Autodesk Inventor part; units mm, degrees
ref_plane "YZ Plane" through (0, 0, 0) normal (1, 0, 0) x (0, 1, 0)
ref_plane "XZ Plane" through (0, 0, 0) normal (0, 1, 0) x (-1, 0, 0)
ref_plane "XY Plane" through (0, 0, 0) normal (0, 0, 1) x (1, 0, 0)
sketch "Sketch1" plane through (0, 0, 0) normal (0, 0, 1) x (1, 0, 0)
  line L0 (0, 0) -> (19.05, 0)
  line L1 (19.05, 0) -> (19.05, 19.05)
  line L2 (69.85, 19.05) -> (69.85, 0)
  line L3 (69.85, 0) -> (88.9, 0)
  line L4 (88.9, 0) -> (88.9, 38.1)
  line L5 (88.9, 38.1) -> (66.675, 57.15)
  line L6 (66.675, 57.15) -> (22.225, 57.15)
  line L7 (22.225, 57.15) -> (0, 38.1)
  line L8 (0, 38.1) -> (0, 0)
  arc A0 (69.85, 19.05) -> (19.05, 19.05) centre (44.45, 19.05) ccw
  dimension "d0" = 38.1
  dimension "d1" = 44.45
  dimension "d2" = 88.9
  dimension "d3" = 19.05
  dimension "d5" = 19.05
  dimension "d6" = 19.05
extrude "Extrusion1" add sketch "Sketch1" against normal blind 127
sketch "Sketch2" plane through (22.225, 57.15, 0) normal (0, 1, 0) x (1, 0, 0)
  line L0 (-22.225, 19.05) -> (68.7148, 19.05)
  line L1 (-22.225, 0) -> (-22.225, 127)
  line L2 (-22.225, 107.95) -> (68.7148, 107.95)
  line L3 (68.7148, 107.95) -> (68.7148, 19.05)
  line L4 (-22.225, 19.05) -> (-22.225, 107.95)
  line L5 (44.45, 0) -> (0, 0)
  line L6 (0, 127) -> (44.45, 127)
  dimension "d9" = 19.05
  dimension "d10" = 19.05
extrude "Extrusion2" cut sketch "Sketch2" against normal through all
sketch "Sketch3" plane through (88.9, 0, 0) normal (1, 0, 0) x (0, 0, -1)
  point P0 (0, 0)
sketch "Sketch4" plane through (88.9, 0, 0) normal (1, 0, 0) x (0, 0, -1)
  line L0 (0, 57.15) -> (0, 88.9)
  line L1 (25.4, 88.9) -> (25.4, 76.2)
  line L2 (25.4, 76.2) -> (101.6, 76.2)
  line L3 (101.6, 76.2) -> (101.6, 88.9)
  line L4 (101.6, 88.9) -> (127, 88.9)
  line L5 (127, 88.9) -> (127, 57.15)
  line L6 (127, 57.15) -> (0, 57.15)
  arc A0 (25.4, 88.9) -> (0, 88.9) centre (12.7, 88.9) ccw
  circle A1 centre (12.7, 88.9) radius 6.35
  point P0 (0, 0)
  dimension "d13" = 31.75
  dimension "d14" = 25.4
  dimension "d15" = 12.7
  dimension "d17" = 12.7
extrude "Extrusion3" add sketch "Sketch4" against normal blind 88.9
sketch "Sketch5" plane through (0, 0, 0) normal (0, 0, 1) x (1, 0, 0)
  line L0 (22.225, 104.8309) -> (22.225, 46.8186)
  line L1 (66.675, 46.8186) -> (66.6601, 105.2632)
  line L2 (0, 57.15) -> (0, 88.9)
  line L3 (22.225, 104.8309) -> (0, 104.8309)
  line L4 (0, 104.8309) -> (0, 57.15)
  line L5 (22.225, 57.15) -> (22.225, 104.8309)
  line L6 (66.6601, 105.2632) -> (88.8851, 105.2632)
  line L7 (88.8851, 105.2632) -> (88.8851, 57.15)
  line L8 (88.8851, 57.15) -> (66.675, 57.15)
  line L9 (0, 57.15) -> (22.225, 57.15)
  line L10 (22.225, 57.15) -> (0, 57.15)
  line L11 (88.9, 57.15) -> (66.675, 57.15)
  line L12 (66.6601, 105.2632) -> (88.9, 105.2632)
  line L13 (88.9, 105.2632) -> (88.9, 57.15)
  line L14 (88.9, 57.15) -> (66.6601, 57.15)
  line L15 (66.6601, 57.15) -> (66.6601, 105.2632)
  point P0 (0, 0)
  dimension "d20" = 22.225
  dimension "d21" = 44.45
extrude "Extrusion4" cut sketch "Sketch5" against normal through all
sketch "Sketch6" plane through (0, 0, 0) normal (0, 0, 1) x (1, 0, 0)
  line L0 (66.6601, 57.15) -> (22.225, 57.15)
  line L1 (34.925, 57.15) -> (34.925, 106.1689)
  line L2 (34.925, 106.1689) -> (53.975, 106.1689)
  line L3 (53.975, 106.1689) -> (53.975, 57.15)
  line L4 (22.225, 88.9) -> (22.225, 57.15)
  point P0 (0, 0)
  dimension "d24" = 19.05
  dimension "d25" = 12.7
extrude "Extrusion5" cut sketch "Sketch6" against normal through all
properties part number "HW 4 Part 4" material "Iron, Cast"
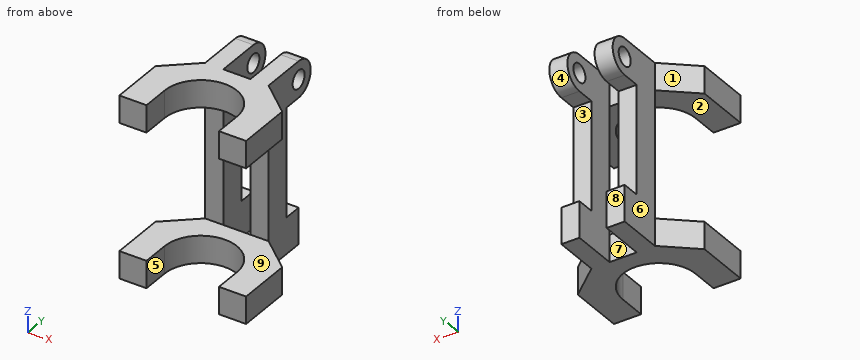
Work out the finished part from the listing and answer in its coordinate system (mm). Face numbers are marked on the shaded views. A direction names the side the tool comes from. Give positions to 0.01 mm unless a question says otherwise; leave off trailing zeros. Loops run counter-clockwise (first coordinate to the right, second up) from the corner with the lowest first, then second, coordinate; pieces in that order, holes last. Notation, with made-up numbers: (39.5, -28.5) -> (66.5, -28.5) arc R13 cw to (66.5, -9.5) -> close; hole circle Ø6 at (45, -33.75). An arc over 180 degrees is marked (long way). Put each result on its own line as item: value. Start each with the question number.
Item 1: The part is cut by section A-A (x = 44.45). Give the vertices of the cut face in (y, z), then the cut area to 3 significant figures.
Item 2: The part is cut by section D-D (y = 40). Give the vertices of the cut face in (x, z).
Item 3: The part is cut by section C-C (y = 74). Give the vertices of the cut face in (x, z) (3 decimals).
Item 4: Each of these flat-tipped pins is pushed along its axis until it touches: P1, Ø3, axis at x = 36, y = 40.5, coming from the +Z side; P2, Ø5, axis at y = 58, z = -108.5, coming from the -X side; P3, Ø1, axis at x = 63, z = -89.5, coming from the +Y side; P4, Ø3, axis at y = 70, z = -70, coming from the +X side. Where does it stop, or does it pass through?
Item 5: The mould has two halves that part along Z. Classify the marked faces 1, 2, 3 and 4: released by +Z, released by -Z, zero draft, split by the parting line, or undercut.
Item 6: The part is cut by section B-B (z = -12.7). Give the vertices of the cut face in (x, y) (3 decimals).
Item 7: Find the intervals of material crossed by L1, parallel to X at y = 92, z = -6.5 (3 decimals); L2, parallel to Z at x = 85, y = 16.5; L3, parallel to Z at x = 57, y = 88, in increasing order. Write a range as [from, to].
Item 8: Which of the six approach directions +Z, -Z, +X, -X, +Y, -Y give full straight-line access (tool end or side, diameter ignored) to the marked faces 5, 6, 7, 8 and 9?
Answers below:
1. outline: (44.45, -127) -> (57.15, -127) -> (57.15, -107.95) -> (44.45, -107.95) -> close; (44.45, -19.05) -> (57.15, -19.05) -> (57.15, 0) -> (44.45, 0) -> close
1. area: 484 mm2
2. outline: (2.22, -127) -> (30.09, -127) -> (30.09, -107.95) -> (2.22, -107.95) -> close; (2.22, -19.05) -> (30.09, -19.05) -> (30.09, 0) -> (2.22, 0) -> close; (58.81, -127) -> (86.68, -127) -> (86.68, -107.95) -> (58.81, -107.95) -> close; (58.81, -19.05) -> (86.68, -19.05) -> (86.68, 0) -> (58.81, 0) -> close
3. outline: (22.225, -127) -> (34.925, -127) -> (34.925, 0) -> (22.225, 0) -> close; (53.975, -127) -> (66.66, -127) -> (66.66, 0) -> (53.975, 0) -> close
4. P1: through
4. P2: x = 20.3
4. P3: y = 76.2
4. P4: x = 66.66
5. face 1: zero draft
5. face 2: undercut
5. face 3: undercut
5. face 4: split by the parting line
6. outline: (0, 0) -> (19.05, 0) -> (19.05, 19.05) arc R25.4 cw to (69.85, 19.05) -> (69.85, 0) -> (88.9, 0) -> (88.9, 38.1) -> (66.675, 57.15) -> (66.66, 57.15) -> (66.66, 82.55) -> (53.975, 82.55) -> (53.975, 57.15) -> (34.925, 57.15) -> (34.925, 82.55) -> (22.225, 82.55) -> (22.225, 57.15) -> (0, 38.1) -> close; (22.225, 95.25) -> (34.925, 95.25) -> (34.925, 101.6) -> (22.225, 101.6) -> close; (53.975, 95.25) -> (66.66, 95.25) -> (66.66, 101.6) -> (53.975, 101.6) -> close
7. L1: [22.225, 34.925], [53.975, 66.66]
7. L2: [-127, -107.95], [-19.05, 0]
7. L3: [-127, -101.6], [-25.4, -18.99], [-6.41, 0]
8. face 5: +Z, -Z, -Y
8. face 6: +Z, -Z, -X, +Y
8. face 7: +Z, -Z, +Y
8. face 8: -Z, +X, -X, +Y
8. face 9: +X, -X, -Y
